Design review of the part built by this model. Coordinates are the model's own, in mm. Give positions to 0.01 mm unless a question says otherwise; leave off trailing zeros. Order: outer loops, then holes, each group sorted by start corner. A loop starts at its lowest first (then second) coordinate and runs counter-clockwise, first axis right, second up. Notation, with made-up numbers: M -39,-5 L -26,-5 A23 ccw -26,9 Z; hole C 34.25,42.5 d5. An arc over 180 degrees is marked long. Put each result on its own line as item: value. Start each with the question number.
from build123d import *

# Parameters (mm, degrees)
BOSS_EXTRUDE1_DEPTH = 4.78
SKETCH3_R           = 4.05
CUT_EXTRUDE1_DEPTH  = 4.78
CIRPATTERN1_COUNT   = 6
CIRPATTERN3_COUNT   = 4


with BuildPart() as part:
    # Sketch2 → Boss-Extrude1 (new body)
    with BuildSketch(Plane(origin=(0, 0, 0), x_dir=(1, 0, 0), z_dir=(0, 1, 0))):
        Polygon((120.740728286, 32.352380638), (88.388347648, 88.388347648), (32.352380638, 120.740728286), (-32.352380638, 120.740728286), (-88.388347648, 88.388347648), (-120.740728286, 32.352380638), (-120.740728286, -32.352380638), (-88.388347648, -88.388347648), (-32.352380638, -120.740728286), (32.352380638, -120.740728286), (88.388347648, -88.388347648), (120.740728286, -32.352380638), align=None)
    extrude(amount=BOSS_EXTRUDE1_DEPTH)

    # Sketch3 → Cut-Extrude1 (cut)
    with BuildSketch(Plane(origin=(0, 4.78, 0), x_dir=(1, 0, 0), z_dir=(0, 1, 0))):
        with Locations(Location((-0.002380638, -105.740728286, 0), (0, 0, 270))):
            Circle(SKETCH3_R)
        with Locations(Location((-0.002380638, -90.740728286, 0), (0, 0, 270))):
            Circle(SKETCH3_R)
    cut_extrude1 = extrude(amount=-CUT_EXTRUDE1_DEPTH, mode=Mode.SUBTRACT)

    # CirPattern1: Cut-Extrude1 ×6 about axis
    cirpattern1_axis = Axis((5.246e-06, 0, -0.216469196), (0, 1, 0))
    for i in range(1, CIRPATTERN1_COUNT):
        add(cut_extrude1.rotate(cirpattern1_axis, i * 360 / CIRPATTERN1_COUNT), mode=Mode.SUBTRACT)

    # CirPattern3: Cut-Extrude1 ×4 about axis
    cirpattern3_axis = Axis((-7e-08, 0, 0.002893764), (0, 1, 0))
    for i in range(1, CIRPATTERN3_COUNT):
        add(cut_extrude1.rotate(cirpattern3_axis, i * 360 / CIRPATTERN3_COUNT), mode=Mode.SUBTRACT)


solid = part.part
1. The part is to be moulded in two halves that separate along X. For faces 1 (the flat face through (-2, 4.78, -2)), 2 (the cylindrical face through (-86.69, 2.42, 0.18)), 3 (the flat face through (104.34, 2.36, 60.76)), 4 (the cylindrical face through (0.176, 2.423, 86.695)), say which applies: +X half, -X half, draft (parallel to the pull), parting line (faces both ways), or undercut.
2. Consider section A-A on x = 79. Give the boundary of the cut face in (y, z), then the cut area to 4 significant figures.
3. Consider section B-B on y = 1.6. Give the number of separate pieces and of enclosed holes in the cut face, then the cut area to 3 significant figures.
4. To check wall thickness, follow probe 1 along X at (y, z) = (1.6, 108); probe 2 along X at (y, z) = (1.7, -106); probe 3 along Z at (x, y) = (102, 1.15). State the ranges of each line that lie inside material, in increasing order.
5. Insertion check: pin 1 (5 mm diameter, centred on x = 0, z = 105.74, fed in from -Y); pin 2 (1.5 mm diameter, centred on y = 2.5, z = -67.5, fed in from -X); pin 3 (2 mm diameter, centred on x = 84, y = 1, fed in from -Z). Each pin has a flat end and moves straight along its axis. Give the tip position at first contact, or say it passes through.
6. Consider section C-C on z = 82.5. Give the boundary of the cut face in (x, y), then the cut area to 3 significant figures.
Returned:
1. face 1: draft
1. face 2: undercut
1. face 3: +X half
1. face 4: undercut
2. outline: M 0,-93.81 L 4.78,-93.81 L 4.78,-49.74 L 0,-49.74 Z; M 0,-41.65 L 4.78,-41.65 L 4.78,41.22 L 0,41.22 Z; M 0,49.31 L 4.78,49.31 L 4.78,93.81 L 0,93.81 Z
2. area: 819.5 mm2
3. separate pieces: 1
3. enclosed holes: 16
3. area: 46,000 mm2
4. probe 1: x = -54.42 to -3.36, 3.36 to 54.42
4. probe 2: x = -57.88 to -4.04, 4.05 to 57.88
4. probe 3: z = -64.81 to -1.55, 1.56 to 64.81
5. pin 1: passes through
5. pin 2: stops at x = -100.88
5. pin 3: stops at z = -91.5
6. outline: M -91.79,0 L 91.79,0 L 91.79,4.78 L -91.79,4.78 Z
6. area: 877 mm2
